Answer from the drawing. Dimensions are ordinates in mm from the lowest x, y and z of the part. A direction names the side the tool comes from. Round coordinates to 2 decimals unless told otherwise and drop trailing zeros. Order: outer loops, then holes, each group sorted by start corner. A loop starts at its lowest first (then second) coordinate and runs counter-clockwise, first axis right, second up. Notation, with made-up numbers: (-15.5, -1.75) -> (14.5, -1.75) arc R11 ccw to (14.5, 15.25) -> close; hole circle Ø9 at (69, 65). An arc over 180 degrees is marked (long way). Use a Markdown table: item, result. Add a question column.
Item 1: Find the intervals of material crossed by L1, parallel to Y at x = 20, z = 24; L2, parallel to X at y = 300, z = 20; L3, parallel to Z at x = 24.5, y = 177, in increasing order. Write a range as [from, to].
Item 2: A cutting plane is placed at A-A, the plane x = 20. Determine the outline of the cut face in (y, z), plus the area to 3 significant figures.
Item 3: A cutting plane is placed at D-D, the plane y = 197.5. Determine the outline of the cut face in (x, z), plus the area to 3 significant figures.
Item 4: A tool of negligible diameter and unlimited length cuts with its end or side. For the marked faces 1, 2, 3 and 4, from which of +Z, -Z, +X, -X, +Y, -Y can it reach the whole face along a straight path? Write none if from no direction.
Item 5: Flat-ended cylindrical pins translate along their axes: P1, Ø1, axis at y = 236, z = 11, coming from the -X side; P2, Ø10, axis at y = 129.5, z = 21, coming from the +X side; P3, Ø3, axis at x = 18, z = 16, coming from the -Y side; P4, Ø1, axis at y = 78.5, z = 8.5, coming from the -X side. Find the tip coordinate at first contact, or state that the pin passes through.
Item 6: A cutting plane is placed at B-B, the plane y = 300. Determine the outline of the cut face in (x, z), plus the area to 3 significant figures.
Item 7: A cutting plane is placed at C-C, the plane z = 14. Determine the outline of the cut face in (x, y), plus the area to 3 significant figures.
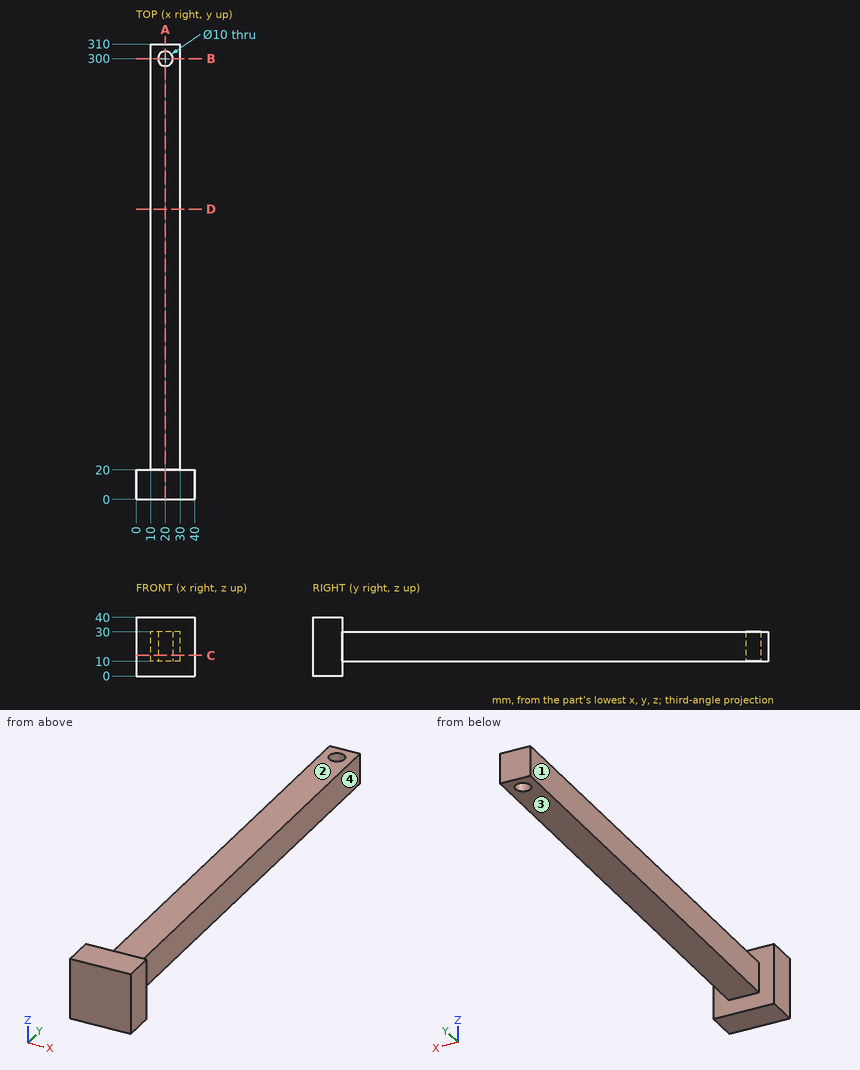
Reported:
| question | item | result |
|---|---|---|
| 1 | L1 | [0, 295], [305, 310] |
| 1 | L2 | [10, 15], [25, 30] |
| 1 | L3 | [10, 30] |
| 2 | outline | (0, 0) -> (20, 0) -> (20, 10) -> (295, 10) -> (295, 30) -> (20, 30) -> (20, 40) -> (0, 40) -> close; (305, 10) -> (310, 10) -> (310, 30) -> (305, 30) -> close |
| 2 | area | 6,400 mm² |
| 3 | outline | (10, 10) -> (30, 10) -> (30, 30) -> (10, 30) -> close |
| 3 | area | 400 mm² |
| 4 | face 1 | +Z, -Z, -X, +Y |
| 4 | face 2 | +Z, +X, -X, +Y |
| 4 | face 3 | -Z, +X, -X, +Y |
| 4 | face 4 | +Z, -Z, +X, +Y |
| 5 | P1 | x = 10 |
| 5 | P2 | x = 30 |
| 5 | P3 | y = 0 |
| 5 | P4 | through |
| 6 | outline | (10, 10) -> (15, 10) -> (15, 30) -> (10, 30) -> close; (25, 10) -> (30, 10) -> (30, 30) -> (25, 30) -> close |
| 6 | area | 200 mm² |
| 7 | outline | (0, 0) -> (40, 0) -> (40, 20) -> (30, 20) -> (30, 310) -> (10, 310) -> (10, 20) -> (0, 20) -> close; hole circle Ø10 at (20, 300) |
| 7 | area | 6,520 mm² |
